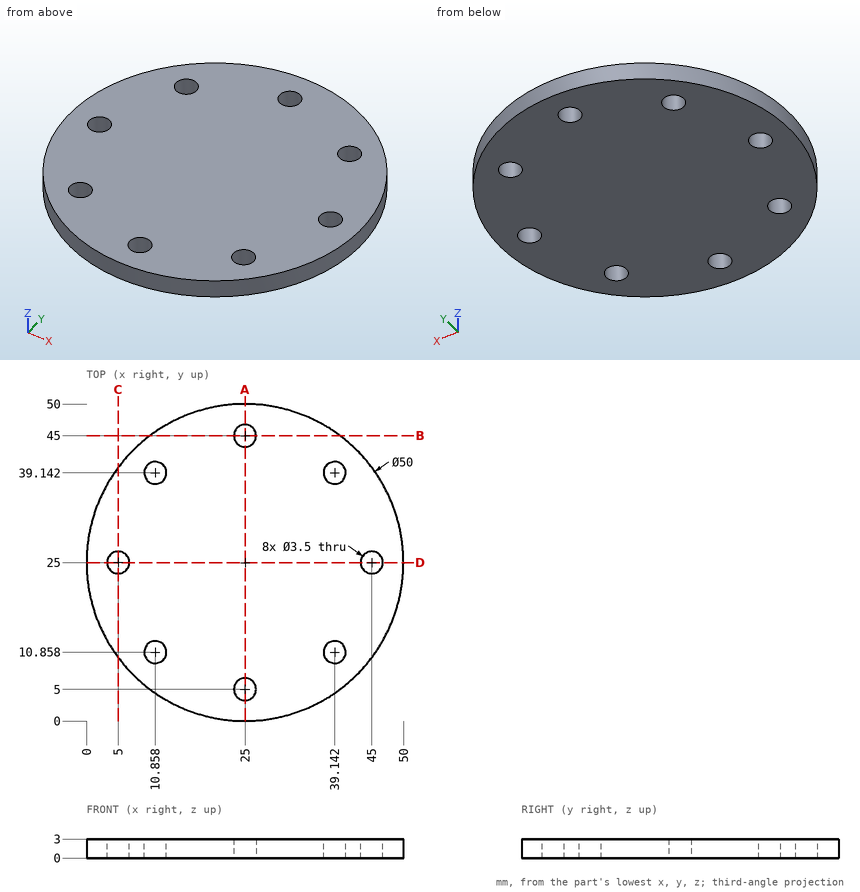
Part print with two shaded views. Sizes in mm from the minimum x, y, z corner. Round coordinates to 2 decimals unless told otherwise and drop trailing zeros. Order: outer loops, then holes, each group sorted by start corner. A loop starts at its lowest first (then second) coordinate and runs counter-clockwise, first axis right, second up. Notation, with made-up numbers: (-8.75, 23) -> (13.25, 23) arc R18 cw to (13.25, 48) -> close; hole circle Ø7 at (2, 3.5). An arc over 180 degrees is marked (long way). Write each question's results on one line, items separated by ' | '.
1. Cut at B-B (y = 45). Give the cut face in (x, z).
Findings below:
outline: (10, 0) -> (23.25, 0) -> (23.25, 3) -> (10, 3) -> close; (26.75, 0) -> (40, 0) -> (40, 3) -> (26.75, 3) -> close
2. Flat gauge pins, fed straight in: P1, Ø1.5, axis at y = 44, z = 0.5, coming from the -X side; P2, Ø1, axis at x = 7.5, z = 2, coming from the +Y side. Where does each tip first touch, or does it go through?
Findings below:
P1: stops at x = 7.91 | P2: stops at y = 43.33
3. Cut at A-A (x = 25). Give the cut face in (y, z), plus the area to 3 significant figures.
Findings below:
outline: (0, 0) -> (3.25, 0) -> (3.25, 3) -> (0, 3) -> close; (6.75, 0) -> (43.25, 0) -> (43.25, 3) -> (6.75, 3) -> close; (46.75, 0) -> (50, 0) -> (50, 3) -> (46.75, 3) -> close | area: 129 mm²
4. Wall check: line 1 along Y through (x, z) = (25, 0.7); line 2 along Y through (x, z) = (11, 0.5); line 3 along X through (y, z) = (26, 0.8). Give the ranges that are in metal, low to high. Write a range as [from, to].
Findings below:
line 1: y = [0, 3.25], [6.75, 43.25], [46.75, 50] | line 2: y = [4.29, 9.11], [12.6, 37.4], [40.89, 45.71] | line 3: x = [0.02, 3.56], [6.44, 43.56], [46.44, 49.98]
